Geometry check sheet. Reference: the model listing, model coordinates, mm. A direction names the side the tool comes from. Give positions to 0.01 mm unless a question says otherwise; leave off trailing zeros. Loops run counter-clockwise (first coordinate to the right, second up) from the corner with the lowest first, then second, coordinate; pieces in that order, holes last. Notation, with made-up numbers: (55, -21.5) - (78, -21.5) arc R19 cw to (78, 10.5) - close; hole circle Ø2 at (-34.5, -3.5). An arc over 180 degrees is marked (long way). Write item = value, one per line. Start each with the question number.
from build123d import *

# Parameters (mm, degrees)
F0_R     = 1.917254
F0_R_2   = 1.651
F0_R_3   = 5.715
F1_DEPTH = 5.08


with BuildPart() as f1:
    # F0 (on Top) → F1 (new body)
    with BuildSketch(Plane.XY):
        with BuildLine():
            ThreePointArc((-23.719894, -3.816054), (-17.291451, -0.972636), (-10.32985, 0))
            Line((-10.32985, 0), (17.073956, 0))
            ThreePointArc((17.073956, 0), (22.687581, 1.659287), (18.118341, 5.318259))
            Line((18.118341, 5.318259), (-10.32985, 5.318259))
            ThreePointArc((-10.32985, 5.318259), (-17.291451, 6.290895), (-23.719894, 9.134313))
            ThreePointArc((-23.719894, 9.134313), (-35.356908, 2.659129), (-23.719894, -3.816054))
        make_face()
        with Locations((0, 2.544119)):
            Circle(F0_R, mode=Mode.SUBTRACT)
        with Locations((19.447466, 2.295572)):
            Circle(F0_R_2, mode=Mode.SUBTRACT)
        with Locations((-27.736908, 2.659129)):
            Circle(F0_R_3, mode=Mode.SUBTRACT)
    extrude(amount=F1_DEPTH)


solid = f1.part
1) Release check for a two-part mould opening along Y. For faces 1 (the face through (-22.286, 4.376, 2.504)), 2 (the face through (-9, 3, 5.08)), 3 (the face through (1.03, 4.16, 2.5)), 4 (the face through (4, 5.318, 3)) record: pulls with the +Y half, pulls with the -Y half, needs draft (parallel to the pull), parting line crosses it, or undercut.
2) Cross-section at C-C on y = 7. Enter the section's corners in (x, z).
3) Gauge pin test, flat end, axial feed: P1, Ø1.5, axis at x = 1.5, z = 3, coming from the +Y side. Record the tip position at first contact, or that the pin passes through.
4) Tool access check on faces 5 (the face through (3, 0, 3)), 6 (the face through (-17.196, 6.264, 2.504)), 7 (the face through (-35.354, 2.886, 2.504)). Record the directions out of +Z, -Z, +X, -X, +Y, -Y that give a thin tool (end or side, any length) a straight path to the whole face; none if there is none.
5) Cross-section at D-D on z = 1.5. Enter the section's corners in (x, y) (1 decimal).
6) Cross-section at B-B on y = 1.75. Enter the section's corners in (x, z).
7) Cross-section at A-A on x = 0. Enter the section's corners in (y, z).
8) Material ranges on line 1 along Y through (x, z) = (0, 3.4); line 2 along Y through (x, z) = (-27.5, 3.5); line 3 along X through (y, z) = (3, 4.65), recorded low to high.
Checked values:
q1.face_1 = undercut
q1.face_2 = needs draft
q1.face_3 = undercut
q1.face_4 = pulls with the +Y half
q2.outline = (-34, 0) - (-31.45, 0) - (-31.45, 5.08) - (-34, 5.08) - close; (-24.02, 0) - (-19.42, 0) - (-19.42, 5.08) - (-24.02, 5.08) - close
q3.P1 = 5.32
q4.face_5 = +Z, -Z, -Y
q4.face_6 = +Z, -Z, +Y
q4.face_7 = +Z, -Z
q5.outline = (-23.7, -3.8) arc R25.4 cw to (-10.3, 0) - (17.1, 0) arc R3.3 ccw (long way) to (18.1, 5.3) - (-10.3, 5.3) arc R25.4 cw to (-23.7, 9.1) arc R7.6 ccw (long way) to start; hole circle Ø11.4 at (-27.7, 2.7); hole circle Ø3.8 at (0, 2.5); hole circle Ø3.3 at (19.4, 2.3)
q6.outline = (-35.3, 0) - (-33.38, 0) - (-33.38, 5.08) - (-35.3, 5.08) - close; (-22.09, 0) - (-1.75, 0) - (-1.75, 5.08) - (-22.09, 5.08) - close; (1.75, 0) - (17.89, 0) - (17.89, 5.08) - (1.75, 5.08) - close; (21.01, 0) - (22.7, 0) - (22.7, 5.08) - (21.01, 5.08) - close
q7.outline = (0, 0) - (0.63, 0) - (0.63, 5.08) - (0, 5.08) - close; (4.46, 0) - (5.32, 0) - (5.32, 5.08) - (4.46, 5.08) - close
q8.line_1 = 0 to 0.63, 4.46 to 5.32
q8.line_2 = -4.96 to -3.05, 8.37 to 10.28
q8.line_3 = -35.35 to -33.44, -22.03 to -1.86, 1.86 to 17.95, 20.94 to 22.67
